from build123d import *

# Parameters (mm, degrees)
CORTE_EXTRUS_O3_REACH         = 16
ESBO_O4_R                     = 7.5
ESBO_O4_R_2                   = 3.25
RESSALTO_EXTRUS_O1_DEPTH      = 2
RESSALTO_EXTRUS_O1_DEPTH_BACK = 7


with BuildPart() as part:
    # Esboço1 → Revolução1 (revolve)
    with BuildSketch(Plane.XY):
        Polygon((3.25, 14), (3.25, 11.5), (5, 11.5), (5, 9), (20, 9), (20, 14), align=None)
    revolve(axis=Axis((0, 0, 0), (0, 1, 0)))

    # Esboço2 → Corte-extrusão3 (cut, up to next)
    with BuildSketch(Plane(origin=(0, 0, 0), x_dir=(1, 0, 0), z_dir=(0, 1, 0)), mode=Mode.PRIVATE) as corte_extrus_o3_sk1:
        with BuildLine():
            ThreePointArc((4.226182617, 9.06307787), (2.164396139, 9.762960071), (0, 10))
            ThreePointArc((0, 10), (-1.5, 11.5), (0, 13))
            ThreePointArc((0, 13), (2.813714981, 12.691848093), (5.494037403, 11.782001231))
            ThreePointArc((5.494037403, 11.782001231), (6.219571691, 9.788612158), (4.226182617, 9.06307787))
        make_face()
    corte_extrus_o3_tool1 = extrude(corte_extrus_o3_sk1.sketch, amount=CORTE_EXTRUS_O3_REACH, mode=Mode.PRIVATE) & part.part
    add(corte_extrus_o3_tool1.solids().sort_by_distance((2.456799, 0, -11.081905))[0], mode=Mode.SUBTRACT)

    # Esboço4 → Ressalto-extrusão1 (add, two sides)
    with BuildSketch(Plane(origin=(0, 14, 0), x_dir=(1, 0, 0), z_dir=(0, 1, 0))) as ressalto_extrus_o1_sk:
        Circle(ESBO_O4_R)
        Circle(ESBO_O4_R_2, mode=Mode.SUBTRACT)
    extrude(amount=RESSALTO_EXTRUS_O1_DEPTH)
    extrude(ressalto_extrus_o1_sk.sketch, amount=-RESSALTO_EXTRUS_O1_DEPTH_BACK)


solid = part.part
Model file for the job. Use its own axes, mm. A direction names the side the tool comes from. Give positions to 0.01 mm unless a question says otherwise; leave off trailing zeros. Loops run counter-clockwise (first coordinate to the right, second up) from the corner with the lowest first, then second, coordinate; pieces in that order, holes last.
Item 1: Drop flat-ended pins along their axis: P1, Ø3, axis at x = 15.5, z = 5, coming from the +Y side; P2, Ø10.5, axis at x = 0, z = 0, coming from the +Y side; P3, Ø1.5, axis at y = 12.5, z = -15.5, coming from the +X side; P4, Ø1, axis at y = 10, z = 9.5, coming from the +X side. Give the stop position or say it passes through.
Check values:
P1: stops at y = 14
P2: stops at y = 16
P3: stops at x = 13.51
P4: stops at x = 17.86
Item 2: Slice it at D-D (z = 4). Write the cut outline in (x, y).
Check values:
outline: (-19.6, 9) - (-6.34, 9) - (-6.34, 7) - (6.34, 7) - (6.34, 9) - (19.6, 9) - (19.6, 14) - (6.34, 14) - (6.34, 16) - (-6.34, 16) - (-6.34, 14) - (-19.6, 14) - close
Item 3: Slice it at A-A (z = 0). Write the cut outline in (x, y), plus the area to 4 significant figures.
Check values:
outline: (-20, 9) - (-7.5, 9) - (-7.5, 7) - (-3.25, 7) - (-3.25, 16) - (-7.5, 16) - (-7.5, 14) - (-20, 14) - close; (3.25, 7) - (7.5, 7) - (7.5, 9) - (20, 9) - (20, 14) - (7.5, 14) - (7.5, 16) - (3.25, 16) - close
area: 201.5 mm2
Item 4: Slice it at B-B (x = 2.5). Write the cut outline in (y, z), plus the area to 3 significant figures.
Check values:
outline: (7, -7.07) - (9, -7.07) - (9, -9.68) - (14, -9.68) - (14, -7.07) - (16, -7.07) - (16, -2.08) - (7, -2.08) - close; (7, 2.08) - (16, 2.08) - (16, 7.07) - (14, 7.07) - (14, 19.84) - (9, 19.84) - (9, 7.07) - (7, 7.07) - close; (9, -19.84) - (14, -19.84) - (14, -12.76) - (9, -12.76) - close
area: 202 mm2
Item 5: Which spindle directions (+Z, -Z, +X, -X, +Y, -Y) get a long thin tool onto all of the face, cutting with end or side? Do faces 1 (the face through (-1.5, 11.5, -11.5)), 2 (the face through (0, 14, 9)), 3 (the face through (2, 16, 3)), 4 (the face through (0, 9, 9)). Say none if no direction does.
Check values:
face 1: +Y, -Y
face 2: +Y
face 3: +Z, -Z, +X, -X, +Y
face 4: -Y
Item 6: Mould opens along Z. For faces 5 (the face through (2.77, 11.46, -12.7)), 6 (the face through (2, 7, 3)), 7 (the face through (-7.493, 8.014, -0.33)) say: +Z half, -Z half, draft (parallel to the pull), parting line (faces both ways), or undercut.
Check values:
face 5: undercut
face 6: draft
face 7: parting line
Item 7: Slice it at C-C (y = 13.25). Write the cut outline in (x, z).
Check values:
outline: circle Ø40 at (0, 0); hole circle Ø6.5 at (0, 0); hole (0, -13) arc R13 ccw to (5.49, -11.78) arc R1.5 ccw to (4.23, -9.06) arc R10 cw to (0, -10) arc R1.5 ccw to start
Item 8: Drill centre lines: line 1 along Z through (x, y) = (0, 14.45); line 2 along X through (y, z) = (9.8, 0). Where is each one in solid material? Low to high.
Check values:
line 1: z = -7.5 to -3.25, 3.25 to 7.5
line 2: x = -20 to -3.25, 3.25 to 20
